Part print with two shaded views. Sizes in mm from the minimum x, y, z corner. A direction names the side the tool comes from. Coordinates: 2 decimals unless noted, no trailing zeros. Loops run counter-clockwise (first coordinate to the right, second up) from the corner with the lowest first, then second, coordinate; pieces in that order, holes last. Notation, with made-up numbers: (-10, 50) -> (49, 50) arc R34 ccw to (49, 88) -> close; hole circle Ø2 at (-29.75, -29). An arc over 180 degrees is marked (long way). Use one line per item in the form item = value.
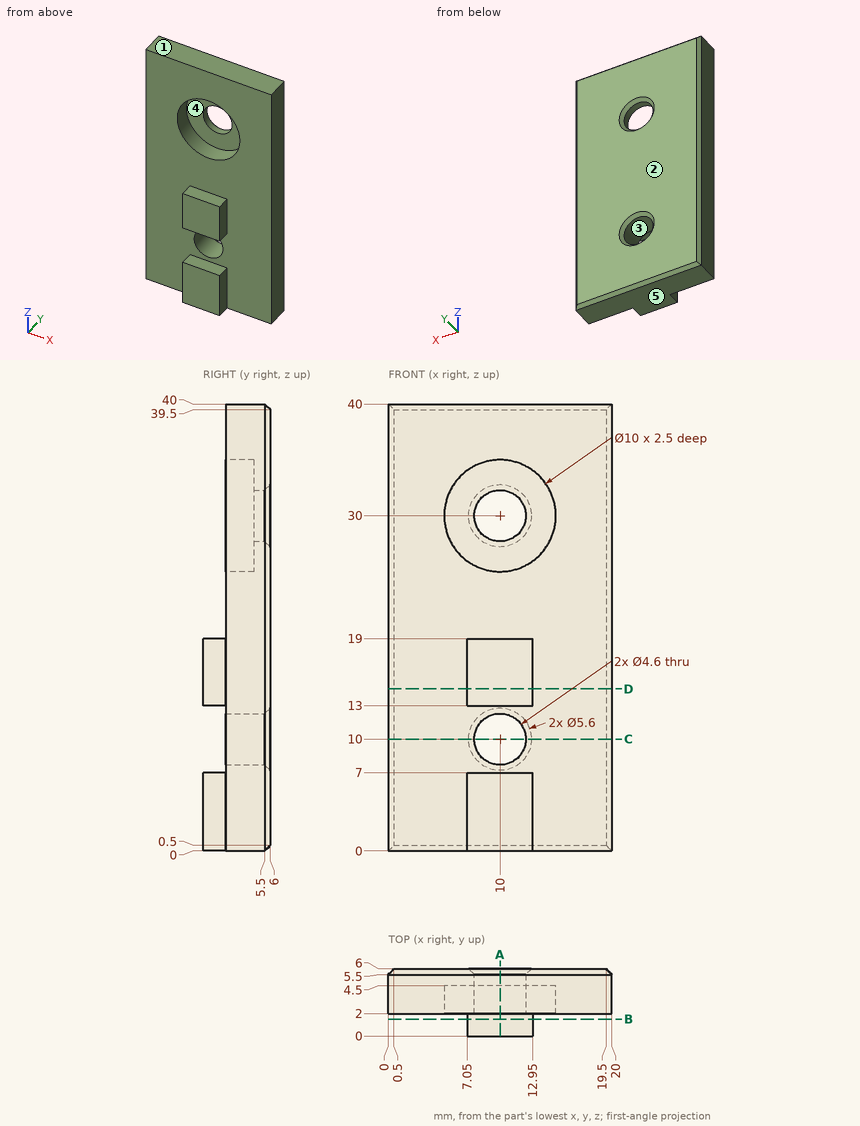
Q1. Band-saw the part on B-B, the plane y = 1.5. Write the cut outline in (x, z).
Result:
outline = (7.05, 0) -> (12.95, 0) -> (12.95, 7) -> (7.05, 7) -> close; (7.05, 13) -> (12.95, 13) -> (12.95, 19) -> (7.05, 19) -> close
Q2. Band-saw the part on A-A, the plane x = 10. Write the cut outline in (y, z).
Result:
outline = (0, 0) -> (5.5, 0) -> (6, 0.5) -> (6, 7.2) -> (5.5, 7.7) -> (2, 7.7) -> (2, 7) -> (0, 7) -> close; (0, 13) -> (2, 13) -> (2, 12.3) -> (5.5, 12.3) -> (6, 12.8) -> (6, 27.2) -> (5.5, 27.7) -> (4.5, 27.7) -> (4.5, 25) -> (2, 25) -> (2, 19) -> (0, 19) -> close; (2, 35) -> (4.5, 35) -> (4.5, 32.3) -> (5.5, 32.3) -> (6, 32.8) -> (6, 39.5) -> (5.5, 40) -> (2, 40) -> close
Q3. Wall check: line 1 along Z through (x, y) = (10, 4.7); line 2 along Z through (x, y) = (10, 3.8); line 3 along X through (y, z) = (4, 10). Give the ranges that are in metal, low to high.
Result:
line_1 = 0 to 7.7, 12.3 to 27.7, 32.3 to 40
line_2 = 0 to 7.7, 12.3 to 25, 35 to 40
line_3 = 0 to 7.7, 12.3 to 20
Q4. Mould opens along Z. For the marked faces 1, 2 and 3 say: released by +Z, released by -Z, zero draft, split by the parting line, or undercut.
Result:
face_1 = released by +Z
face_2 = zero draft
face_3 = undercut
Q5. Band-saw the part on C-C, the plane z = 10. Write the cut outline in (x, y), and give its area (3 significant figures).
Result:
outline = (0, 2) -> (7.7, 2) -> (7.7, 5.5) -> (7.2, 6) -> (0.5, 6) -> (0, 5.5) -> close; (12.3, 2) -> (20, 2) -> (20, 5.5) -> (19.5, 6) -> (12.8, 6) -> (12.3, 5.5) -> close
area = 61.1 mm2
Q6. Which spindle directions (+Z, -Z, +X, -X, +Y, -Y) get a long thin tool onto all of the face, cutting with end or side? Do the marked faces 4 and 5. Say none if no direction does.
Result:
face_4 = -Y
face_5 = -Z, +X, -X, +Y, -Y
Q7. Pin check, flat tips, straight feed: pin 1 Ø2 at (x, y) = (10, 2.5) entering from -Z; pin 2 Ø2 at (y, z) = (0.5, 4) entering from -X; pin 3 Ø0.6 at (x, y) = (10, 1) entering from +Z; pin 4 Ø3 at (x, z) = (12, 29) entering from -Y. Stop position of each tip, or through.
Result:
pin_1 = 0
pin_2 = 7.05
pin_3 = 19
pin_4 = 4.5
Q8. Band-saw the part on D-D, the plane z = 14.5. Write the cut outline in (x, y), and give its area (4 significant figures).
Result:
outline = (0, 2) -> (7.05, 2) -> (7.05, 0) -> (12.95, 0) -> (12.95, 2) -> (20, 2) -> (20, 5.5) -> (19.5, 6) -> (0.5, 6) -> (0, 5.5) -> close
area = 91.55 mm2
